Part model, mm, in its own coordinate system. Round coordinates to 2 decimals unless told otherwise and drop trailing zeros. Write each loop counter-clockwise with the first axis right and the second up, starting at its lowest first coordinate (ties: lowest second). Pieces come first, ordered by that corner, then holes. Notation, with made-up numbers: M -11,59.5 L 47,59.5 A17 cw 47,86.5 Z; hole C 15.25,-17 d3. An arc over 180 degrees is marked long. Use one line per item in the form item = value. Start each with the question number.
Item 1: Cut at C-C, the plane x = 18.5. Give the cut face in (y, z), then the cut area to 3 significant figures.
Item 2: Cut at B-B, the plane y = 1. State how many separate pieces and enclosed holes the cut face has, then the cut area to 3 significant figures.
Item 3: Probe L1, parallel to Z at x = 10.85, y = 3.2; L2, parallel to X at y = 0.35, z = -1; L3, parallel to Z at x = -25.4, y = 4.4. List the from-to ranges inside material, lowest first.
Item 4: Flat gauge pin, fed straight in: pin 1 Ø1.5 at (x, z) = (-18, -5) entering from -Y. Where does the tip first touch, or does it go through?
Item 5: Cut at A-A, the plane x = 27. Give the cut face in (y, z).
Item 6: Mould opens along X. For faces 1 (the face through (25.82, 2.96, -40.42)), 2 (the face through (-28.97, 3.04, -40.65)), 3 (the face through (0, 3, -42.15)) say: +X half, -X half, draft (parallel to the pull), parting line (faces both ways), or undercut.
from build123d import *

# Parameters (mm, degrees)
BOSS_EXTRUDE1_DEPTH         = 6
FILLET1_R                   = 5
F_24_0_152_DIAMETER_HOLE1_D = 3.8608
F_0_257_DIAMETER_HOLE1_D    = 6.5278


with BuildPart() as part:
    # Sketch1 → Boss-Extrude1 (new body)
    with BuildSketch(Plane(origin=(0, 0, 0), x_dir=(1, 0, 0), z_dir=(0, 1, 0))):
        Polygon((-9, -42.15), (-30.4, -23.364405734), (-30.4, 42.15), (30.4, 42.15), (30.4, -23.364405734), (9, -42.15), align=None)
    extrude(amount=BOSS_EXTRUDE1_DEPTH)

    # Fillet1
    fillet1_edges = [part.edges().sort_by_distance(p)[0] for p in [
        (-30.4, 3, -42.15),
        (30.4, 3, -42.15),
        (30.4, 3, 23.364405734),
        (-30.4, 3, 23.364405734),
    ]]
    fillet(fillet1_edges, radius=FILLET1_R)

    # #24 (0.152) Diameter Hole1 (through all)
    with Locations(Plane(origin=(0, 6, 0), x_dir=(1, 0, 0), z_dir=(0, 1, 0))):
        with Locations((10.85, -0.325), (-10.85, -0.325), (-10.85, 31.425), (10.85, 31.425), (12.5, -34.65), (-12.5, -34.65)):
            Hole(F_24_0_152_DIAMETER_HOLE1_D / 2)

    # F (0.257) Diameter Hole1 (through all)
    with Locations(Plane(origin=(0, 6, 0), x_dir=(1, 0, 0), z_dir=(0, 1, 0))):
        with Locations((25.4, 37.185), (-25.4, 37.185), (-25.4, -13.615), (25.4, -13.615)):
            Hole(F_0_257_DIAMETER_HOLE1_D / 2)


solid = part.part
Model answer:
q1.outline = M 0,-42.15 L 6,-42.15 L 6,33.81 L 0,33.81 Z
q1.area = 456 mm²
q2.separate_pieces = 1
q2.enclosed_holes = 10
q2.area = 4,510 mm²
q3.L1 = -42.15 to -33.36, -29.49 to -1.61, 2.26 to 33.65, 35.65 to 40.53
q3.L2 = -30.4 to -12.25, -9.45 to 9.45, 12.25 to 30.4
q3.L3 = -42.15 to -40.45, -33.92 to 10.35, 16.88 to 27.75
q4.pin_1 = 0
q5.outline = M 0,-41.89 L 6,-41.89 L 6,-40.03 L 0,-40.03 Z; M 0,-34.34 L 6,-34.34 L 6,10.77 L 0,10.77 Z; M 0,16.46 L 6,16.46 L 6,26.35 L 0,26.35 Z
q6.face_1 = undercut
q6.face_2 = -X half
q6.face_3 = draft
